The model under review builds one solid part; all positions refer to its coordinate system, in mm. Coordinates: 2 decimals unless noted, no trailing zeros. Write each loop counter-clockwise with the first axis right and the second up, starting at its lowest first coordinate (ties: lowest second). Pieces come first, ordered by that corner, then holes. Notation, with made-up numbers: (42.25, 5) - (64.25, 5) arc R20 cw to (64.25, 14) - close; hole circle Ø5 at (33, 68). An arc over 180 degrees is marked (long way). Return JSON: item names as keys, results as strings. Group by question number.
(1) We need section A-A on y = -25. State the section outline as (x, z) points.
(2) For pin 1 Ø3.5 at (x, y) = (-15, -15) entering from -Z, flat-tipped, find the tip position at first contact; note if it passes through.
(3) We need section C-C on z = 0.15. Give the number of separate pieces and of enclosed holes in the cut face, then the cut area to 3 significant figures.
(4) To check wall thickness, follow L1, parallel to Y at x = -25, z = 0.3; L2, parallel to X at y = -5.5, z = 0.4; L3, parallel to X at y = -3.5, z = 0.4. State the ranges of each line that lie inside material, in increasing order. Write a range as from..to.
Autodesk Inventor part; units mm, degrees
ref_plane "YZ Plane" through (0, 0, 0) normal (1, 0, 0) x (0, 1, 0)
ref_plane "XZ Plane" through (0, 0, 0) normal (0, 1, 0) x (-1, 0, 0)
ref_plane "XY Plane" through (0, 0, 0) normal (0, 0, 1) x (1, 0, 0)
sketch "Náčrt1" plane through (0, 0, 0) normal (0, 0, 1) x (1, 0, 0)
  line L0 (-40, 10) -> (10, 10)
  line L1 (10, 10) -> (10, -40)
  line L2 (10, -40) -> (-40, -40)
  line L3 (-40, -40) -> (-40, 10)
  point P0 (0, 0)
  dimension "d0" = 50
  dimension "d1" = 50
  dimension "d2" = 10
  dimension "d3" = 10
extrude "Vysunutí1" add sketch "Náčrt1" along normal blind 0.5
sketch "Náčrt2" plane through (0, 0, 0.5) normal (0, 0, 1) x (1, 0, 0)
  circle A0 centre (-35, 5) radius 2
  line L0 (10, 10) -> (-40, 10)
  line L1 (-40, 10) -> (-40, -40)
  point P0 (0, 0)
  dimension "d6" = 4
  dimension "d7" = 5
  dimension "d8" = 5
extrude "Vysunutí2" cut sketch "Náčrt2" against normal blind 0.5
pattern_linear "Obdélníkové pole1" count 5 spacing 10 along (1, 0, 0) count 5 spacing 10 along (0, -1, 0) of "Vysunutí2"
fillet "Zaoblení1" radius 1 1 edges at (10, 10, 0.25)
fillet "Zaoblení2" radius 1 2 edges at (-40, 10, 0.25) (-40, -40, 0.25)
fillet "Zaoblení3" radius 1 1 edges at (10, -40, 0.25)
properties part number "1072"
Ans:
{
 "1": {"outline": "(-40, 0) - (-37, 0) - (-37, 0.5) - (-40, 0.5) - close; (-33, 0) - (-27, 0) - (-27, 0.5) - (-33, 0.5) - close; (-23, 0) - (-17, 0) - (-17, 0.5) - (-23, 0.5) - close; (-13, 0) - (-7, 0) - (-7, 0.5) - (-13, 0.5) - close; (-3, 0) - (3, 0) - (3, 0.5) - (-3, 0.5) - close; (7, 0) - (10, 0) - (10, 0.5) - (7, 0.5) - close"},
 "2": {"pin 1": "through"},
 "3": {"separate pieces": "1", "enclosed holes": "25", "area": "2,180 mm²"},
 "4": {"L1": "-40..-37, -33..-27, -23..-17, -13..-7, -3..3, 7..10", "L2": "-40..-36.94, -33.06..-26.94, -23.06..-16.94, -13.06..-6.94, -3.06..3.06, 6.94..10", "L3": "-40..-36.32, -33.68..-26.32, -23.68..-16.32, -13.68..-6.32, -3.68..3.68, 6.32..10"}
}
